Here's how the part is built. I have some questions about the finished solid (model axes, mm). Round coordinates to 2 decimals unless told otherwise and drop trailing zeros. Order: outer loops, then holes, each group sorted by start corner. A loop starts at its lowest first (then second) coordinate and runs counter-clockwise, first axis right, second up. Notation, with made-up numbers: (-16.5, 55.5) -> (10.5, 55.5) arc R25 ccw to (10.5, 69.5) -> close; hole circle Ø4 at (54, 60). An arc over 180 degrees is marked (long way). One line per item, written item: value.
Autodesk Inventor part; units mm, degrees
ref_plane "YZ Plane" through (0, 0, 0) normal (1, 0, 0) x (0, 1, 0)
ref_plane "XZ Plane" through (0, 0, 0) normal (0, 1, 0) x (-1, 0, 0)
ref_plane "XY Plane" through (0, 0, 0) normal (0, 0, 1) x (1, 0, 0)
sketch "Sketch1" plane through (0, 0, 0) normal (0, 1, 0) x (-1, 0, 0)
  line L0 (0, 0) -> (94, 0)
  line L1 (94, -100) -> (0, -100)
  line L2 (0, -100) -> (0, 0)
  line L3 (94, 0) -> (0, 0) construction
  line L4 (0, 0) -> (0, -9) construction
  line L5 (0, -9) -> (94, -9) construction
  line L6 (94, -9) -> (94, 0) construction
  line L7 (0, -100) -> (94, -100) construction
  line L8 (94, -100) -> (94, -91) construction
  line L9 (94, -91) -> (0, -91) construction
  line L10 (0, -91) -> (0, -100) construction
  line L11 (94, 0) -> (94, -100)
  circle A0 centre (78.3333, -6) radius 1.6
  circle A1 centre (15.6667, -6) radius 1.6
  circle A2 centre (78.3333, -94) radius 1.6
  circle A3 centre (15.6667, -94) radius 1.6
  line L12 (82.3582, -14) -> (7, -80.7604)
  line L13 (7, -80.7604) -> (7, -14)
  line L14 (7, -14) -> (82.3582, -14)
  line L15 (87, -19.2396) -> (11.6418, -86)
  line L16 (11.6418, -86) -> (87, -86)
  line L17 (87, -86) -> (87, -19.2396)
  line L18 (82.3582, -14) -> (87, -19.2396) construction
  line L19 (11.6418, -86) -> (7, -80.7604) construction
  dimension "d0" = 100
  dimension "d1" = 9
  dimension "d2" = 3
  dimension "d3" = 3.2
  dimension "d4" = 15.6667
  dimension "d5" = 62.6667
  dimension "d6" = 94
  dimension "d7" = 3
  dimension "d10" = 7
  dimension "d11" = 7
  dimension "d12" = 7
  dimension "d13" = 5
  dimension "d14" = 5
extrude "Extrusion1" add sketch "Sketch1" along normal blind 3
fillet "Fillet1" radius 3 6 edges at (-82.3582, 1.5, -14) (-7, 1.5, -14) (-7, 1.5, -80.7604) (-87, 1.5, -19.2396) (-11.6418, 1.5, -86) (-87, 1.5, -86)
equation "\"d4\" = 0.166667 * d6"
equation "\"d5\" = 4 * d4"
equation "\"d11\" = d10"
equation "\"d12\" = d11"
equation "\"d14\" = d13"
properties part number "FrontPanel"
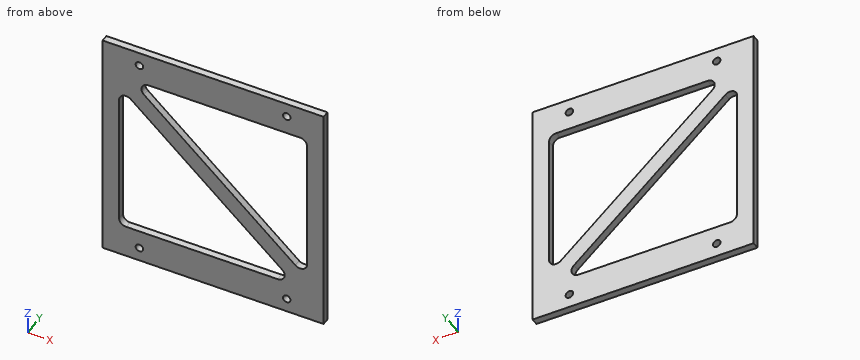
Q1. I need wall thicknesses on line 1 along X through (y, z) = (1.2, -94); line 2 along Z through (x, y) = (-15.5, 0.2); line 3 along Z through (x, y) = (-20, 0.3). Which ranges of each line are inside material? Lowest first, please.
Answers:
line 1: -94 to -79.93, -76.73 to -17.27, -14.07 to 0
line 2: -100 to -95.59, -92.41 to -73.23, -14 to -7.59, -4.41 to 0
line 3: -100 to -86, -78.6 to -69.24, -14 to 0
Q2. For P1, Ø1.9, axis at x = -78.33, z = -6, coming from the -Y side, with a flat end and sliding along its axis, tell me the tip position at first contact or that it passes through.
Answers:
P1: through
Q3. I want a section at A-A on y = 2. Write out the boundary of the cut face in (x, z).
Answers:
outline: (-94, -100) -> (0, -100) -> (0, 0) -> (-94, 0) -> close; hole (-87, -83) arc R3 ccw to (-84, -86) -> (-19.55, -86) arc R3 ccw to (-17.56, -80.75) -> (-82.01, -23.66) arc R3 ccw to (-87, -25.91) -> close; hole circle Ø3.2 at (-78.33, -94); hole circle Ø3.2 at (-78.33, -6); hole (-76.44, -19.25) -> (-11.99, -76.34) arc R3 ccw to (-7, -74.09) -> (-7, -17) arc R3 ccw to (-10, -14) -> (-74.45, -14) arc R3 ccw to start; hole circle Ø3.2 at (-15.67, -94); hole circle Ø3.2 at (-15.67, -6)
Q4. I want a section at C-C on x = -56. Write out the boundary of the cut face in (y, z).
Answers:
outline: (0, -100) -> (3, -100) -> (3, -86) -> (0, -86) -> close; (0, -46.7) -> (3, -46.7) -> (3, -37.35) -> (0, -37.35) -> close; (0, -14) -> (3, -14) -> (3, 0) -> (0, 0) -> close
Q5. I want a section at B-B on z = -6. Write out the boundary of the cut face in (x, y), then the cut area to 3 significant figures.
Answers:
outline: (-94, 0) -> (-79.93, 0) -> (-79.93, 3) -> (-94, 3) -> close; (-76.73, 0) -> (-17.27, 0) -> (-17.27, 3) -> (-76.73, 3) -> close; (-14.07, 0) -> (0, 0) -> (0, 3) -> (-14.07, 3) -> close
area: 263 mm2
